from build123d import *

# Parameters (mm, degrees)
SKETCH1_W               = 60
SKETCH1_H               = 72
BOTTOM_DEPTH            = 2
SKETCH2_R               = 2.25
PIN_LOCS_DEPTH          = 4
SKETCH5_R               = 1.25
PIN_HOLES_DEPTH         = 4
SKETCH3_R               = 2.25
SKETCH3_R_2             = 2.15
SENSOR_PINS_DEPTH       = 8
SKETCH6_R               = 1.25
SKETCH6_R_2             = 1.2
PIN_HOLES_SENSORS_DEPTH = 4
SKETCH4_W               = 8
SKETCH4_H               = 10
POWER_CABLE_DEPTH       = 2
SKETCH7_W               = 16.5
SKETCH7_H               = 25
SKETCH7_W_2             = 17
SKETCH7_H_2             = 13
SKETCH7_W_3             = 15.833991833
SKETCH7_W_4             = 13.166008167
SKETCH7_W_5             = 15.5
CUT_EXTRUDE1_DEPTH      = 2


with BuildPart() as part:
    # Sketch1 → Bottom (new body)
    with BuildSketch(Plane(origin=(0, 0, 0), x_dir=(1, 0, 0), z_dir=(0, 1, 0))):
        Rectangle(SKETCH1_W, SKETCH1_H)
    extrude(amount=BOTTOM_DEPTH)

    # Sketch2 → Pin Locs (add)
    with BuildSketch(Plane(origin=(0, 2, 0), x_dir=(1, 0, 0), z_dir=(0, 1, 0))):
        with Locations(Location((25.7, -13.1, 0), (0, 0, 90))):
            Circle(SKETCH2_R)
        with Locations(Location((-20.7, -13.1, 0), (0, 0, 270))):
            Circle(SKETCH2_R)
        with Locations(Location((25.7, -31.5, 0), (0, 0, 270))):
            Circle(SKETCH2_R)
        with Locations(Location((-20.7, -31.5, 0), (0, 0, 90))):
            Circle(SKETCH2_R)
    extrude(amount=PIN_LOCS_DEPTH)

    # Sketch5 → Pin Holes (cut)
    with BuildSketch(Plane(origin=(0, 6, 0), x_dir=(1, 0, 0), z_dir=(0, 1, 0))):
        with Locations(Location((-20.7, -31.5, 0), (0, 0, 270))):
            Circle(SKETCH5_R)
        with Locations(Location((-20.7, -13.1, 0), (0, 0, 270))):
            Circle(SKETCH5_R)
        with Locations(Location((25.7, -13.1, 0), (0, 0, 270))):
            Circle(SKETCH5_R)
        with Locations(Location((25.7, -31.5, 0), (0, 0, 270))):
            Circle(SKETCH5_R)
    extrude(amount=-PIN_HOLES_DEPTH, mode=Mode.SUBTRACT)

    # Sketch3 → Sensor Pins (add)
    with BuildSketch(Plane(origin=(0, 2, 0), x_dir=(1, 0, 0), z_dir=(0, 1, 0))):
        with Locations(Location((20.7, 19.7, 0), (0, 0, 270))):
            Circle(SKETCH3_R)
        with Locations(Location((20.7, -1.2, 0), (0, 0, 90))):
            Circle(SKETCH3_R)
        with Locations(Location((7.5, -1.2, 0), (0, 0, 270))):
            Circle(SKETCH3_R)
        with Locations(Location((7.5, 19.7, 0), (0, 0, 90))):
            Circle(SKETCH3_R)
        with Locations(Location((-1.1, 19.7, 0), (0, 0, 270))):
            Circle(SKETCH3_R_2)
        with Locations(Location((-1.1, -1.2, 0), (0, 0, 90))):
            Circle(SKETCH3_R_2)
        with Locations(Location((-14.3, -1.2, 0), (0, 0, 270))):
            Circle(SKETCH3_R_2)
        with Locations(Location((-14.3, 19.7, 0), (0, 0, 90))):
            Circle(SKETCH3_R_2)
    extrude(amount=SENSOR_PINS_DEPTH)

    # Sketch6 → Pin Holes Sensors (cut)
    with BuildSketch(Plane(origin=(0, 10, 0), x_dir=(1, 0, 0), z_dir=(0, 1, 0))):
        with Locations(Location((-14.3, -1.2, 0), (0, 0, 270))):
            Circle(SKETCH6_R)
        with Locations(Location((-1.1, -1.2, 0), (0, 0, 270))):
            Circle(SKETCH6_R)
        with Locations(Location((-1.1, 19.7, 0), (0, 0, 270))):
            Circle(SKETCH6_R_2)
        with Locations(Location((-14.3, 19.7, 0), (0, 0, 270))):
            Circle(SKETCH6_R_2)
        with Locations(Location((20.7, -1.2, 0), (0, 0, 270))):
            Circle(SKETCH6_R_2)
        with Locations(Location((20.7, 19.7, 0), (0, 0, 270))):
            Circle(SKETCH6_R_2)
    extrude(amount=-PIN_HOLES_SENSORS_DEPTH, mode=Mode.SUBTRACT)

    # Sketch4 → Power Cable (cut)
    with BuildSketch(Plane(origin=(0, 2, 0), x_dir=(1, 0, 0), z_dir=(0, 1, 0))):
        with Locations((26, 31)):
            Rectangle(SKETCH4_W, SKETCH4_H)
    extrude(amount=-POWER_CABLE_DEPTH, mode=Mode.SUBTRACT)

    # Sketch7 → Cut-Extrude1 (cut)
    with BuildSketch(Plane(origin=(0, 2, 0), x_dir=(1, 0, 0), z_dir=(0, 1, 0))):
        with Locations((-7.75, -20.5)):
            Rectangle(SKETCH7_W, SKETCH7_H)
        with Locations((-18.5, 9.5)):
            Rectangle(SKETCH7_W_2, SKETCH7_H_2)
        with Locations((1.916995917, 9.5)):
            Rectangle(SKETCH7_W_3, SKETCH7_H_2)
        with Locations((20.416995916, 9.5)):
            Rectangle(SKETCH7_W_4, SKETCH7_H_2)
        with Locations((12.25, -20.5)):
            Rectangle(SKETCH7_W_5, SKETCH7_H)
    extrude(amount=-CUT_EXTRUDE1_DEPTH, mode=Mode.SUBTRACT)


solid = part.part
Read the model definition and answer for the solid it produces. Units are mm, in the model's axes. A direction names the side the tool comes from. Give positions to 0.01 mm unless a question says otherwise; leave off trailing zeros. Write each loop counter-clockwise with the first axis right and the second up, starting at its lowest first coordinate (ties: lowest second). Pieces come first, ordered by that corner, then holes. Notation, with made-up numbers: (-25.5, 65) - (-6.5, 65) arc R14 cw to (-6.5, 80) - close; hole circle Ø11 at (71.5, -35.75). An arc over 180 degrees is marked (long way). Answer in a Markdown table with one row per item. Add a question column.
Item 1: Section A-A, the plane y = 4 is taken. Count the separate pieces of the cut face and the enclosed holes in it, and give its area (3 significant figures).
Item 2: Section B-B, the plane x = -14.3 is taken. Write down the section's boundary in (y, z).
Item 3: Find the intervals of material crossed by L1, parallel to X at y = 3.1, z = 31.5; L2, parallel to Z at x = -13, y = 1.75; L3, parallel to Z at x = -2, y = 6.25, in increasing order.
Item 4: Section D-D, the plane z = 10 is taken. Write down the section's boundary in (x, y), and give its area (3 significant figures).
Item 5: A tool of negligible diameter and unlimited length cuts with its end or side. For faces 1 (the face through (12, 1, 8)), 2 (the face through (0.208, 5.944, 2.906)), 3 (the face through (22, 10, 0)), from which of +Z, -Z, +X, -X, +Y, -Y can it reach the whole face along a straight path? Write none if from no direction.
Item 6: Determine the mould class of faces 4 (the face through (-19.7, 6, 30.5)), 5 (the face through (-13.06, 8.03, 1.04)) for opening direction Z: pulls with the +Z half, pulls with the -Z half, needs draft (parallel to the pull), parting line crosses it, or undercut.
Item 7: Flat-ended cylindrical pins translate along their axes: P1, Ø4, axis at x = -11.5, z = -14.5, coming from the +Y side; P2, Ø5, axis at x = -12, y = 6.5, coming from the -Z side; P3, Ø1.5, axis at x = 0, y = 5.5, coming from the +Z side. Find the tip coordinate at first contact, or state that the pin passes through.
Recorded:
| question | item | result |
|---|---|---|
| 1 | separate pieces | 12 |
| 1 | enclosed holes | 4 |
| 1 | area | 166 mm2 |
| 2 | outline | (0, -36) - (2, -36) - (2, -21.85) - (10, -21.85) - (10, -20.9) - (6, -20.9) - (6, -18.5) - (10, -18.5) - (10, -17.55) - (2, -17.55) - (2, -16) - (0, -16) - close; (0, -3) - (2, -3) - (2, -0.95) - (10, -0.95) - (10, -0.05) - (6, -0.05) - (6, 2.45) - (10, 2.45) - (10, 3.35) - (2, 3.35) - (2, 8) - (0, 8) - close; (0, 33) - (2, 33) - (2, 36) - (0, 36) - close |
| 3 | L1 | x = -22.95 to -21.95, -19.45 to -18.45, 23.45 to 24.45, 26.95 to 27.95 |
| 3 | L2 | z = -36 to -16, -3 to 8, 33 to 36 |
| 3 | L3 | z = -21.65 to -20.49, -18.91 to -17.75, -0.75 to 0.33, 2.07 to 3.15 |
| 4 | outline | (-30, 0) - (-16, 0) - (-16, 2) - (-30, 2) - close; (0.5, 0) - (4.5, 0) - (4.5, 2) - (0.5, 2) - close; (20, 0) - (30, 0) - (30, 2) - (20, 2) - close |
| 4 | area | 56.0 mm2 |
| 5 | face 1 | +Y, -Y |
| 5 | face 2 | +Y |
| 5 | face 3 | +Z, -Z, +X, -X, +Y |
| 6 | face 4 | needs draft |
| 6 | face 5 | undercut |
| 7 | P1 | stops at y = 2 |
| 7 | P2 | stops at z = -21.85 |
| 7 | P3 | stops at z = 3.32 |
